from build123d import *

# Parameters (mm, degrees)
CUBO_START            = 27.75
SK_CUBO_R             = 23
CUBO_DEPTH            = 19
PASANTES_M4_START     = 27.75
SK_PASANTES_M4_R      = 2.25
PASANTES_M4_DEPTH     = 19
CENTRADOR_D42_START   = 27.75
SK_CENTRADOR_D42_R    = 21.2
CENTRADOR_D42_DEPTH   = 1.2
PASADORES_MOTOR_START = 27.75
SK_PASADORES_MOTOR_R  = 2.6
PASADORES_MOTOR_DEPTH = 5


with BuildPart() as part:
    # Sk_Cubo → Cubo (new body)
    with BuildSketch(Plane(origin=(0, 0, 0), x_dir=(1, 0, 0), z_dir=(0, 1, 0)).offset(CUBO_START)):
        with Locations(Location((0, -170, 0), (0, 0, 270))):
            Circle(SK_CUBO_R)
    extrude(amount=CUBO_DEPTH)

    # Sk_Pasantes_M4 → Pasantes_M4 (cut)
    with BuildSketch(Plane(origin=(0, 0, 0), x_dir=(1, 0, 0), z_dir=(0, 1, 0)).offset(PASANTES_M4_START)):
        with Locations(Location((14.839084994, -167.808754572, 0), (0, 0, 270))):
            Circle(SK_PASANTES_M4_R)
        with Locations(Location((9.317216704, -181.75540186, 0), (0, 0, 270))):
            Circle(SK_PASANTES_M4_R)
        with Locations(Location((-5.52186829, -183.946647288, 0), (0, 0, 270))):
            Circle(SK_PASANTES_M4_R)
        with Locations(Location((-14.839084994, -172.191245428, 0), (0, 0, 270))):
            Circle(SK_PASANTES_M4_R)
        with Locations(Location((-9.317216704, -158.24459814, 0), (0, 0, 270))):
            Circle(SK_PASANTES_M4_R)
        with Locations(Location((5.52186829, -156.053352712, 0), (0, 0, 270))):
            Circle(SK_PASANTES_M4_R)
    extrude(amount=PASANTES_M4_DEPTH, mode=Mode.SUBTRACT)

    # Sk_Centrador_D42 → Centrador_D42 (cut)
    with BuildSketch(Plane(origin=(0, 0, 0), x_dir=(1, 0, 0), z_dir=(0, 1, 0)).offset(CENTRADOR_D42_START)):
        with Locations(Location((0, -170, 0), (0, 0, 270))):
            Circle(SK_CENTRADOR_D42_R)
    extrude(amount=CENTRADOR_D42_DEPTH, mode=Mode.SUBTRACT)

    # Sk_Pasadores_motor → Pasadores_motor (cut)
    with BuildSketch(Plane(origin=(0, 0, 0), x_dir=(1, 0, 0), z_dir=(0, 1, 0)).offset(PASADORES_MOTOR_START)):
        with Locations(Location((13.295803748, -175.264181103, 0), (0, 0, 270))):
            Circle(SK_PASADORES_MOTOR_R)
        with Locations(Location((-11.20681644, -178.882413258, 0), (0, 0, 270))):
            Circle(SK_PASADORES_MOTOR_R)
        with Locations(Location((-2.088987308, -155.853405639, 0), (0, 0, 270))):
            Circle(SK_PASADORES_MOTOR_R)
    extrude(amount=PASADORES_MOTOR_DEPTH, mode=Mode.SUBTRACT)


solid = part.part
The listing builds one solid part. Answer for the finished solid, in the listing's coordinates (mm). A direction names the side the tool comes from. Give positions to 0.01 mm unless a question says otherwise; leave off trailing zeros. Loops run counter-clockwise (first coordinate to the right, second up) from the corner with the lowest first, then second, coordinate; pieces in that order, holes last. Notation, with made-up numbers: (-10.75, -25) - (44.25, -25) arc R16 cw to (44.25, -2) - close; hole circle Ø3 at (2.5, -1). An arc over 180 degrees is marked (long way). Use one line per item in the form item = value.
1. The mould has two halves that part along X. Classify faces 3 (the face through (-2, 32.75, 156)), 4 (the face through (-13, 31, 177)), 5 (the face through (0, 46.75, 170)), 6 (the face through (1.011, 37.117, 147.022)): pulls with the +X half, pulls with the -X half, needs draft (parallel to the pull), parting line crosses it, or undercut.
Calculated:
face_3 = undercut
face_4 = undercut
face_5 = needs draft
face_6 = parting line crosses it
2. Given pin 1 Ø5 at (x, z) = (-5.52, 183.95) entering from -Y; pin 2 Ø4 at (x, y) = (-4, 37) entering from -Z; pin 3 Ø10 at (x, y) = (16, 44) entering from +Z, each flat-ended and moving along its own axis, determine where each tip first touches the part or whether it passes through.
Calculated:
pin_1 = 28.95
pin_2 = 147.09
pin_3 = 190.2
3. Section A-A on z = 173.5 is taken. Give the vertices of the cut face in (x, y).
Calculated:
outline = (-22.73, 27.75) - (-20.91, 27.75) - (-20.91, 28.95) - (-16.67, 28.95) - (-16.67, 46.75) - (-22.73, 46.75) - close; (-13.01, 28.95) - (11.39, 28.95) - (11.39, 32.75) - (15.21, 32.75) - (15.21, 28.95) - (20.91, 28.95) - (20.91, 27.75) - (22.73, 27.75) - (22.73, 46.75) - (-13.01, 46.75) - close
4. Which of the six approach directions +Z, -Z, +X, -X, +Y, -Y give full straight-line access (tool end or side, diameter ignored) to faces 1 (the face through (0, 28.95, 170)), 2 (the face through (-19, 27.75, 180))?
Calculated:
face_1 = -Y
face_2 = +Z, -Z, +X, -X, -Y
5. Find the intervals of material crossed by line 1 along Y through (x, z) = (-1, 170); line 2 along Y through (x, z) = (-12, 180.5); line 3 along X through (y, z) = (37, 168), in increasing order. Write a range as [from, to].
Calculated:
line_1 = [28.95, 46.75]
line_2 = [32.75, 46.75]
line_3 = [-22.91, 12.6], [17.08, 22.91]
6. Section C-C on y = 32 is taken. Count the separate pieces of the cut face and the enclosed holes in it, then the cut area to 3 significant figures.
Calculated:
separate_pieces = 1
enclosed_holes = 9
area = 1,500 mm^2
7. Section D-D on y = 35.75 is taken. Give the vertices of the cut face in (x, z), then the cut area to 3 significant figures.
Calculated:
outline = circle Ø46 at (0, 170); hole circle Ø4.5 at (-14.84, 172.19); hole circle Ø4.5 at (-9.32, 158.24); hole circle Ø4.5 at (-5.52, 183.95); hole circle Ø4.5 at (5.52, 156.05); hole circle Ø4.5 at (9.32, 181.76); hole circle Ø4.5 at (14.84, 167.81)
area = 1,570 mm^2
8. Section B-B on x = 16.5 is taken. Give the vertices of the cut face in (y, z).
Calculated:
outline = (27.75, 153.98) - (46.75, 153.98) - (46.75, 166.29) - (28.95, 166.29) - (28.95, 156.69) - (27.75, 156.69) - close; (27.75, 183.31) - (28.95, 183.31) - (28.95, 169.33) - (46.75, 169.33) - (46.75, 186.02) - (27.75, 186.02) - close
